Check sheet for the modelled part. Datum: model origin and axes. Units: mm. Face numbers are marked on the shaded views. A direction names the side the tool comes from. Round coordinates to 2 decimals unless told otherwise and drop trailing zeros. Loops run counter-clockwise (first coordinate to the right, second up) from the corner with the lowest first, then second, coordinate; pieces in that order, holes last. Notation, with made-up numbers: (-38, 84) -> (-8, 84) arc R20 ccw to (-8, 105) -> close; hole circle Ø2 at (29, 79). An arc over 180 degrees is marked (long way). One line per question, with ' | ' between items.
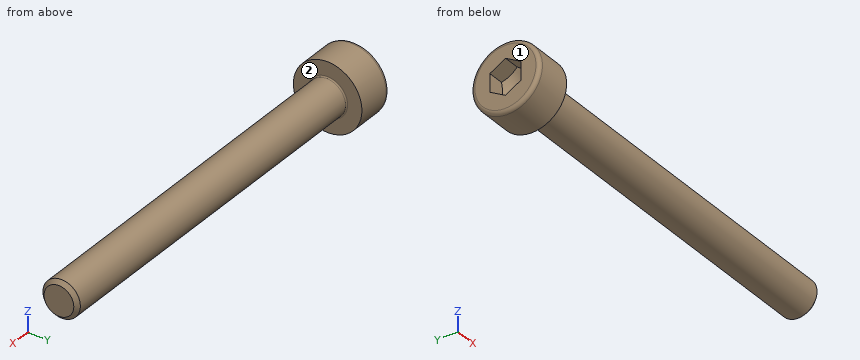
Autodesk Inventor part; units mm, degrees
ref_plane "Work Plane1" through (29, 0, 0) normal (0, -1, 0) x (1, 0, 0)
ref_plane "YZ Plane" through (0, 0, 0) normal (1, 0, 0) x (0, 1, 0)
ref_plane "XZ Plane" through (0, 0, 0) normal (0, 1, 0) x (-1, 0, 0)
sketch "Sketch1" plane through (0, 0, 0) normal (0, 0, 1) x (1, 0, 0)
  line L0 (-0.8667, 0) -> (30, 0)
  line L1 (30, 0) -> (30, 1.5)
  line L2 (30, 1.5) -> (23.25, 1.5)
  line L3 (23.25, 1.5) -> (22.9432, 1.5)
  line L4 (22.9432, 1.5) -> (0, 1.5)
  line L5 (0, 1.5) -> (0, 2.75)
  line L6 (0, 2.75) -> (-3, 2.75)
  line L7 (-3, 2.75) -> (-3, 1.4434)
  line L8 (-3, 1.4434) -> (-1.7, 1.4434)
  line L9 (-1.7, 1.4434) -> (-0.8667, 0)
  line L10 (-9.6, 0) -> (36.6, 0)
  line L11 (0, -0.55) -> (0, 3.3)
  line L12 (23.25, 1.5) -> (0, 1.5) construction
  dimension "d1" = 6.75
  dimension "d2" = 0.3068
  dimension "d3" = 3
  dimension "d4" = 1.3
  dimension "d5" = 60
  dimension "d6" = 3
  dimension "d7" = 3
  dimension "d8" = 2.8868
  dimension "d9" = 5.5
  dimension "d26" = 30
revolve "Body" add sketch "Sketch1" angle 360 about axis through (-0.8667, 0, 0) along (1, 0, 0)
sketch "Sketch2" plane through (-3, 0, 0) normal (-1, 0, 0) x (0, 0, 1)
  circle A0 centre (0, 0) radius 1.4434
  line L0 (0, -3.85) -> (0, 3.85)
  line L1 (-3.85, 0) -> (3.85, 0)
  line L2 (1.4434, 0) -> (0.7217, -1.25)
  line L3 (0.7217, -1.25) -> (-0.7217, -1.25)
  line L4 (-0.7217, -1.25) -> (-1.4434, 0)
  line L5 (-1.4434, 0) -> (-0.7217, 1.25)
  line L6 (-0.7217, 1.25) -> (0.7217, 1.25)
  line L7 (0.7217, 1.25) -> (1.4434, 0)
extrude "Slot" add sketch "Sketch2" against normal up to next contours L7 A0 | A0 L2 | L6 L0 A0 | A0 L0 L3 | L0 L6 A0 | A0 L3 L0 | L4 A0 | A0 L5
fillet "Fillet1" radius 0.3 1 edges at (-3, -2.75, 0)
thread "Thread"
chamfer "Chamfer1" distance 0.3067 distance2 0.3067 1 edges at (30, -1.5, 0) measured on face at (30, -0.3888, 0.2119)
ref_plane "Work Plane1" through (29, 0, 0) normal (0, -1, 0) x (1, 0, 0)
fillet "Fillet2" radius 0.1 1 edges at (0, -1.5, 0)
equation "\"d1\" = GEL"
equation "\"d3\" = KOH"
equation "\"d4\" = INTI"
equation "\"d6\" = GD"
equation "\"d7\" = BDM"
equation "\"d8\" = 1.1547 * SW"
equation "\"d9\" = KOD"
equation "\"d17\" = RR"
equation "\"d13\" = GEL"
equation "\"d15\" = -0.5 * SPD + 0.5 * GD"
equation "\"d16\" = GUL"
equation "\"d30\" = R"
equation "\"GD\" = NND"
equation "\"NLG\" = 8"
equation "\"GEL\" = 6.75"
equation "\"KOD\" = 5.5"
equation "\"KOH\" = NND"
equation "\"INTI\" = 1.3"
equation "\"GAL\" = 0.61345 * PTC"
equation "\"GUL\" = 0.61345 * PTC"
equation "\"BDM\" = NND"
equation "\"SW\" = 2.5"
equation "\"RR\" = 0.1 * NND"
equation "\"SPD\" = NND - 1.2269 * PTC"
equation "\"R\" = 0.1"
equation "\"PHH\" = 0.13"
equation "\"GD1\" = THREADDIA - 1.2269 * PTC"
equation "\"THREADDIA\" = 3"
equation "\"FAWI\" = 45deg"
equation "\"PTC\" = 0.5"
equation "\"KOH1\" = 2.7"
equation "\"NND\" = 3"
equation "\"TOA\" = 30deg"
equation "\"E0\" = 1.155 * SW"
properties part number "AS 1420 - 1973 - M3 x 8" material "Steel, Mild"
(1) Go/stop test with flat-tipped pins: pin 1 (2 mm diameter, centred on x = 3, z = 0.5, fed in from -Y); pin 2 (3 mm diameter, centred on x = 6, z = 2, fed in from -Y). Record where each tip stops, or that it passes through.
Answer:
pin 1: stops at y = -1.5 | pin 2: stops at y = -1.41
(2) Scan lines: probe 1 along Y at (x, z) = (27, 0.9); probe 2 along Z at (x, y) = (8.5, 0.1); probe 3 along X at (y, z) = (0.9, 1.45). Record each from-to range of solid material in increasing order.
Answer:
probe 1: y = -1.2 to 1.2 | probe 2: z = -1.5 to 1.5 | probe 3: x = -3 to 0
(3) Set-up check for the marked faces 1 and 2: record each of +Z, -Z, +X, -X, +Y, -Y from which the full face is reachable in a straight line by a thin tool's end or side.
Answer:
face 1: +Z, -Z, -X, +Y, -Y | face 2: +X
(4) Sectioned sample at A-A, the plane x = 8.5. Record the cut outline in (y, z).
Answer:
outline: circle Ø3 at (0, 0)
